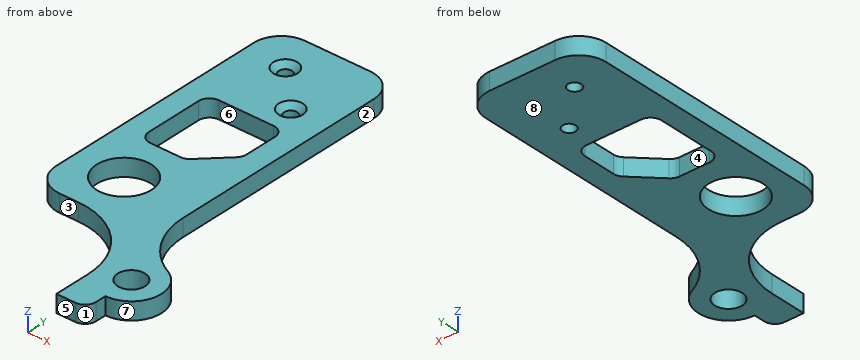
```python
from build123d import *

# Parameters (mm, degrees)
SKETCH1_R                                       = 2.5
SKETCH1_R_2                                     = 5
BOSS_EXTRUDE1_DEPTH                             = 3.175
CSK_FOR_M2_FLAT_HEAD_MACHINE_SCREW3_D           = 2.4
CSK_FOR_M2_FLAT_HEAD_MACHINE_SCREW3_CSINK_D     = 4.4
CSK_FOR_M2_FLAT_HEAD_MACHINE_SCREW3_CSINK_ANGLE = 90
CUT_EXTRUDE2_DEPTH                              = 68.698453638
F_5MM_FILLET_R                                  = 5
F_2MM_FILLET_R                                  = 2
F_1MM_FILLET_R                                  = 1
CUT_EXTRUDE3_DEPTH                              = 68.698453638
FILLET1_R                                       = 5
BOSS_EXTRUDE2_DEPTH                             = 3.175
BOSS_EXTRUDE3_START                             = -3.175
SKETCH14_W                                      = 5.5
SKETCH14_H                                      = 4
BOSS_EXTRUDE3_DEPTH                             = 3.175
FILLET3_R                                       = 2
CUT_EXTRUDE6_DEPTH                              = 68.698453638
CUT_EXTRUDE6_DEPTH_BACK                         = 10
FILLET6_R                                       = 13
FILLET7_R                                       = 13


with BuildPart() as part:
    # Sketch1 → Boss-Extrude1 (new body)
    with BuildSketch(Plane.XY):
        with BuildLine():
            Line((0, -5.5), (-7, -5.5))
            Line((-7, -5.5), (-7, -9))
            Line((-7, -9), (-12, -9))
            Line((-12, -9), (-12, -2.5))
            Line((-12, -2.5), (-27, 4.494614872))
            Line((-27, 4.494614872), (-27, 62))
            Line((-27, 62), (-5, 62))
            Line((-5, 62), (-5, 32.19632141))
            Line((-5, 32.19632141), (-9, 28.19632141))
            Line((-9, 28.19632141), (-9, 10.265347478))
            Line((-9, 10.265347478), (2.32440044, 4.984692829))
            ThreePointArc((2.32440044, 4.984692829), (5.369628039, -1.190417877), (0, -5.5))
        make_face()
        Circle(SKETCH1_R, mode=Mode.SUBTRACT)
        with Locations((-18, 19.2)):
            Circle(SKETCH1_R_2, mode=Mode.SUBTRACT)
    extrude(amount=BOSS_EXTRUDE1_DEPTH)

    # CSK for M2 Flat Head Machine Screw3 (through all)
    with Locations(Plane.XY.offset(3.175)):
        with Locations((-19.5, 55), (-12, 47.5)):
            CounterSinkHole(CSK_FOR_M2_FLAT_HEAD_MACHINE_SCREW3_D / 2, CSK_FOR_M2_FLAT_HEAD_MACHINE_SCREW3_CSINK_D / 2, counter_sink_angle=CSK_FOR_M2_FLAT_HEAD_MACHINE_SCREW3_CSINK_ANGLE)

    # Sketch11 → Cut-Extrude2 (cut, through all)
    with BuildSketch(Plane.XY.offset(3.175)):
        Polygon((-23, 28.19632141), (-23, 42.69632141), (-9, 42.69632141), (-9, 33.85317566), (-14.65, 28.19632141), align=None)
    extrude(amount=-CUT_EXTRUDE2_DEPTH, mode=Mode.SUBTRACT)

    # 5mm_Fillet
    f_5mm_fillet_edges = [part.edges().sort_by_distance(p)[0] for p in [
        (-12, -2.5, 1.5875),
        (-27, 4.494614872, 1.5875),
        (-27, 62, 1.5875),
        (-5, 62, 1.5875),
        (-5, 32.19632141, 1.5875),
        (-9, 28.19632141, 1.5875),
        (-9, 10.265347478, 1.5875),
    ]]
    fillet(f_5mm_fillet_edges, radius=F_5MM_FILLET_R)

    # 2mm_Fillet
    f_2mm_fillet_edges = [part.edges().sort_by_distance(p)[0] for p in [
        (-14.65, 28.19632141, 1.5875),
        (-23, 28.19632141, 1.5875),
        (-23, 42.69632141, 1.5875),
        (-9, 42.69632141, 1.5875),
        (-9, 33.85317566, 1.5875),
    ]]
    fillet(f_2mm_fillet_edges, radius=F_2MM_FILLET_R)

    # 1mm_Fillet
    f_1mm_fillet_edges = [part.edges().sort_by_distance(p)[0] for p in [
        (-7, -5.5, 1.5875),
        (-7, -9, 1.5875),
    ]]
    fillet(f_1mm_fillet_edges, radius=F_1MM_FILLET_R)

    # Sketch12 → Cut-Extrude3 (cut, through all)
    with BuildSketch(Plane.XY.offset(3.175)):
        with BuildLine():
            Line((-27, 10.199636133), (-27, -4.690363867))
            Line((-27, -4.690363867), (-12.1, -4.690363867))
            Line((-12.1, -4.690363867), (-12.1, 5.199636133))
            ThreePointArc((-12.1, 5.199636133), (-13.564466094, 8.735170039), (-17.1, 10.199636133))
            Line((-17.1, 10.199636133), (-27, 10.199636133))
        make_face()
    extrude(amount=-CUT_EXTRUDE3_DEPTH, mode=Mode.SUBTRACT)

    # Fillet1
    fillet1_edges = [part.edges().sort_by_distance(p)[0] for p in [
        (-27, 10.199636133, 1.5875),
    ]]
    fillet(fillet1_edges, radius=FILLET1_R)

    # Sketch13 → Boss-Extrude2 (add)
    with BuildSketch(Plane.XY.offset(3.175)):
        with BuildLine():
            Line((-5, 34.267389222), (-5, 8.400116845))
            Line((-5, 8.400116845), (-6.113091309, 8.919159847))
            ThreePointArc((-6.113091309, 8.919159847), (-8.216957229, 10.76420074), (-9, 13.450698782))
            Line((-9, 13.450698782), (-9, 26.125253598))
            ThreePointArc((-9, 26.125253598), (-8.619397663, 28.03867076), (-7.535533906, 29.660787504))
            Line((-7.535533906, 29.660787504), (-6.464466094, 30.731855316))
            ThreePointArc((-6.464466094, 30.731855316), (-5.380602337, 32.35397206), (-5, 34.267389222))
        make_face()
    extrude(amount=-BOSS_EXTRUDE2_DEPTH)

    # Sketch14 → Boss-Extrude3 (add)
    with BuildSketch(Plane.XY.offset(3.175).offset(BOSS_EXTRUDE3_START)):
        with Locations((-2.75, -7.5)):
            Rectangle(SKETCH14_W, SKETCH14_H)
        with BuildLine():
            ThreePointArc((0, -5.5), (-3.889087297, -3.889087297), (-5.5, 0))
            Line((-5.5, 0), (-5.5, -5.5))
            Line((-5.5, -5.5), (0, -5.5))
        make_face()
    extrude(amount=BOSS_EXTRUDE3_DEPTH)

    # Fillet3
    fillet3_edges = [part.edges().sort_by_distance(p)[0] for p in [
        (0, -9.5, 1.5875),
    ]]
    fillet(fillet3_edges, radius=FILLET3_R)

    # Sketch15 → Cut-Extrude6 (cut, two sides: drawn at the far end of the back side and taken through both)
    with BuildSketch(Plane.XY.offset(3.175).offset(-CUT_EXTRUDE6_DEPTH_BACK)):
        with BuildLine():
            Line((-5.5, 10.199636133), (-17.1, 10.199636133))
            ThreePointArc((-17.1, 10.199636133), (-13.564466094, 8.735170039), (-12.1, 5.199636133))
            Line((-12.1, 5.199636133), (-12.1, -4.690363867))
            ThreePointArc((-12.1, -4.690363867), (-12.035186912, -5.09321027), (-12.003436692, -5.5))
            Line((-12.003436692, -5.5), (-6, -5.5))
            Line((-6, -5.5), (-5.5, -5.5))
            Line((-5.5, -5.5), (-5.5, 10.199636133))
        make_face()
    extrude(amount=CUT_EXTRUDE6_DEPTH + CUT_EXTRUDE6_DEPTH_BACK, mode=Mode.SUBTRACT)


with BuildPart() as body_2:
    # of the pieces the cut leaves, the one that is kept (cut_extrude6_keep)
    add(part.part.solids().sort_by_distance((0, -7.5, 0))[0])

    # Fillet6
    fillet6_edges = [body_2.edges().sort_by_distance(p)[0] for p in [
        (-5.5, 10.199636133, 1.5875),
    ]]
    fillet(fillet6_edges, radius=FILLET6_R)

    # Fillet7
    fillet7_edges = [body_2.edges().sort_by_distance(p)[0] for p in [
        (-5, 8.400116845, 1.5875),
    ]]
    fillet(fillet7_edges, radius=FILLET7_R)


solid = body_2.part
```
Can you work these out from the model? Positions are in its coordinate system, mm. Face numbers are marked on the shaded views. A direction names the side the tool comes from. Coordinates: 2 decimals unless noted, no trailing zeros. Order: outer loops, then holes, each group sorted by start corner. A loop starts at its lowest first (then second) coordinate and runs counter-clockwise, first axis right, second up.
1. If we section it at C-C (x = -12): Please give me the cut outline in (y, z) (3 decimals).
2. If we section it at A-A (y = 47.5): Please give me the cut outline in (x, z) (3 decimals).
3. For the marked faces 1, 2, 3 and 4, which set-ups out of +Z, -Z, +X, -X, +Y, -Y let a thin tool reach every point of the face, with its end or its side?
4. I'm going to push flat-ended pins straight in: pin 1 (1.6 mm diameter, centred on x = -15.5, z = 2, fed in from -Y); pin 2 (1 mm diameter, centred on y = 38, z = 2, fed in from +X); pin 3 (1.6 mm diameter, centred on y = -7, z = 2.5, fed in from +X); pin 4 (1.9 mm diameter, centred on x = -12, y = 47.5, fed in from +Z). Where does each tip first touch, or does it pass through?
5. Thinking about a two-plate mould opening in Y: for the marked faces 5, 6, 7 and 8, which applies, +Y half, -Y half, draft (parallel to the pull), parting line (faces both ways), or undercut?
6. I need wall thicknesses on line 1 (X direction, y = 19.5, z = 1.2); line 2 (X direction, y = 55, z = 0.9); line 3 (Y direction, x = -19.5, z = 0.6). Which ranges of each line are inside material? Lowest first, please.
7. If we section it at B-B (x = -19.5): Please give me the cut outline in (y, z) (3 decimals).
8. If we section it at D-D (z = 1.5): Give the number of separate pieces and of enclosed holes in the cut face, then the cut area to 3 significant figures.
Entries:
1. outline: (8.458, 0) - (30.85, 0) - (30.85, 3.175) - (8.458, 3.175) - close; (42.696, 0) - (46.3, 0) - (46.3, 2.175) - (45.3, 3.175) - (42.696, 3.175) - close; (48.7, 0) - (62, 0) - (62, 3.175) - (49.7, 3.175) - (48.7, 2.175) - close
2. outline: (-27, 0) - (-13.2, 0) - (-13.2, 2.175) - (-14.2, 3.175) - (-27, 3.175) - close; (-10.8, 0) - (-5, 0) - (-5, 3.175) - (-9.8, 3.175) - (-10.8, 2.175) - close
3. face 1: +Z, -Z, +X, -Y
3. face 2: +Z, -Z, +X, +Y
3. face 3: +Z, -Z, -X, -Y
3. face 4: +Z, -Z
4. pin 1: stops at y = 9.63
4. pin 2: stops at x = -5
4. pin 3: stops at x = 0
4. pin 4: passes through
5. face 5: -Y half
5. face 6: undercut
5. face 7: parting line
5. face 8: draft
6. line 1: x = -27 to -22.99, -13.01 to -5
6. line 2: x = -27 to -20.7, -18.3 to -5
6. line 3: y = 10.2 to 14.43, 23.97 to 28.2, 42.7 to 53.8, 56.2 to 62
7. outline: (10.2, 0) - (14.43, 0) - (14.43, 3.175) - (10.2, 3.175) - close; (23.97, 0) - (28.196, 0) - (28.196, 3.175) - (23.97, 3.175) - close; (42.696, 0) - (53.8, 0) - (53.8, 2.175) - (52.8, 3.175) - (42.696, 3.175) - close; (56.2, 0) - (62, 0) - (62, 3.175) - (57.2, 3.175) - (56.2, 2.175) - close
8. separate pieces: 1
8. enclosed holes: 5
8. area: 1,020 mm2
